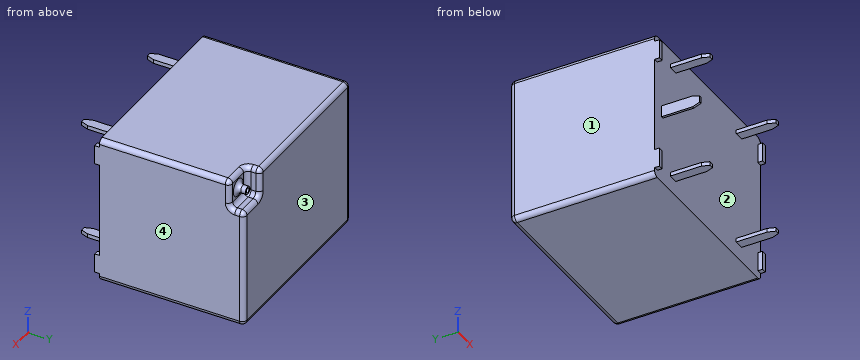
from build123d import *
from OCP.BRepFilletAPI import BRepFilletAPI_MakeChamfer

# Parameters (mm, degrees)
SKETCH_1_W          = 19.6
SKETCH_1_H          = 15.6
EXTRUDE_1_DEPTH     = 15.2
SKETCH_2_W          = 3
SKETCH_2_H          = 3
CUT_EXTRUDE_1_DEPTH = 1.5
SKETCH_3_R          = 0.4
SKETCH_3_R_2        = 0.25
EXTRUDE_2_DEPTH     = 1
SKETCH_5_W          = 0.5
SKETCH_5_H          = 2
EXTRUDE_4_DEPTH     = 0.5
FILLET_1_R          = 0.5
SKETCH_4_W          = 0.25
SKETCH_4_H          = 1.2
SKETCH_4_W_2        = 1
SKETCH_4_H_2        = 0.4
EXTRUDE_3_DEPTH     = 4
CHAMFER_1_SIZE      = 0.75
CHAMFER_1_SIZE2     = 0.272977676


with BuildPart() as part:
    # Эскиз1 → Бобышка-Вытянуть1 (new body)
    with BuildSketch(Plane(origin=(0, 0, 0), x_dir=(1, 0, 0), z_dir=(0, 1, 0))):
        Rectangle(SKETCH_1_W, SKETCH_1_H)
    extrude(amount=EXTRUDE_1_DEPTH)

    # Эскиз2 → Вырез-Вытянуть1 (cut)
    with BuildSketch(Plane(origin=(0, 15.2, 0), x_dir=(1, 0, 0), z_dir=(0, 1, 0))):
        with Locations((8.3, -6.3)):
            Rectangle(SKETCH_2_W, SKETCH_2_H)
    extrude(amount=-CUT_EXTRUDE_1_DEPTH, mode=Mode.SUBTRACT)

    # Эскиз3 → Бобышка-Вытянуть2 (add)
    with BuildSketch(Plane(origin=(0, 13.7, 0), x_dir=(1, 0, 0), z_dir=(0, 1, 0))):
        with Locations(Location((8.3, -6.3, 0), (0, 0, 270))):
            Circle(SKETCH_3_R)
        with Locations(Location((8.3, -6.3, 0), (0, 0, 270))):
            Circle(SKETCH_3_R_2, mode=Mode.SUBTRACT)
    extrude(amount=EXTRUDE_2_DEPTH)

    # Эскиз5 → Бобышка-Вытянуть4 (add)
    with BuildSketch(Plane.XZ):
        with Locations((-9.55, 6)):
            Rectangle(SKETCH_5_W, SKETCH_5_H)
        with Locations((-9.55, -6)):
            Rectangle(SKETCH_5_W, SKETCH_5_H)
        with Locations((9.55, -6)):
            Rectangle(SKETCH_5_W, SKETCH_5_H)
        with Locations((9.55, 6)):
            Rectangle(SKETCH_5_W, SKETCH_5_H)
    extrude(amount=EXTRUDE_4_DEPTH)

    # Скругление1
    fillet_1_edges = [part.edges().sort_by_distance(p)[0] for p in [
        (8.3, 15.2, 4.8),
        (-9.8, 7.6, -7.8),
        (-9.8, 15.2, 0),
        (9.8, 7.6, -7.8),
        (0, 15.2, -7.8),
        (9.8, 15.2, -1.5),
        (8.3, 13.7, 5.9),
        (6.8, 13.7, 6.3),
        (8.3, 13.7, 4.8),
        (9.8, 14.45, 4.8),
        (8.3, 13.7, 7.8),
        (9.8, 13.7, 6.3),
        (6.8, 14.45, 4.8),
        (6.8, 15.2, 6.3),
        (6.8, 14.45, 7.8),
        (-1.5, 15.2, 7.8),
        (9.8, 6.85, 7.8),
        (-9.8, 7.6, 7.8),
    ]]
    fillet(fillet_1_edges, radius=FILLET_1_R)

    # Эскиз4 → Бобышка-Вытянуть3 (add)
    with BuildSketch(Plane.XZ):
        with Locations((-8.4, 0)):
            Rectangle(SKETCH_4_W, SKETCH_4_H)
        with Locations((-6.4, 6)):
            Rectangle(SKETCH_4_W_2, SKETCH_4_H_2)
        with Locations((5.8, 6)):
            Rectangle(SKETCH_4_W_2, SKETCH_4_H_2)
        with Locations((5.8, -6)):
            Rectangle(SKETCH_4_W_2, SKETCH_4_H_2)
        with Locations((-6.4, -6)):
            Rectangle(SKETCH_4_W_2, SKETCH_4_H_2)
    extrude(amount=EXTRUDE_3_DEPTH)

    # Фаска1: one chamfer whose edges measure the first distance from different faces: ONE call of the kernel's chamfer builder (chamfer() names one face for all edges)
    chamfer_1_edges_1 = [part.edges().sort_by_distance(p)[0] for p in [
        (-8.4, -4, 0.6),
    ]]
    chamfer_1_side_1 = [part.faces().sort_by_distance(p)[0] for p in [
        (-8.4, -2, 0.6),
    ]]
    chamfer_1_edges_2 = [part.edges().sort_by_distance(p)[0] for p in [
        (-8.4, -4, -0.6),
    ]]
    chamfer_1_side_2 = [part.faces().sort_by_distance(p)[0] for p in [
        (-8.4, -2, -0.6),
    ]]
    chamfer_1_edges_3 = [part.edges().sort_by_distance(p)[0] for p in [
        (-6.9, -4, 6),
    ]]
    chamfer_1_side_3 = [part.faces().sort_by_distance(p)[0] for p in [
        (-6.9, -2, 6),
    ]]
    chamfer_1_edges_4 = [part.edges().sort_by_distance(p)[0] for p in [
        (-5.9, -4, 6),
    ]]
    chamfer_1_side_4 = [part.faces().sort_by_distance(p)[0] for p in [
        (-5.9, -2, 6),
    ]]
    chamfer_1_edges_5 = [part.edges().sort_by_distance(p)[0] for p in [
        (5.3, -4, 6),
    ]]
    chamfer_1_side_5 = [part.faces().sort_by_distance(p)[0] for p in [
        (5.3, -2, 6),
    ]]
    chamfer_1_edges_6 = [part.edges().sort_by_distance(p)[0] for p in [
        (6.3, -4, 6),
    ]]
    chamfer_1_side_6 = [part.faces().sort_by_distance(p)[0] for p in [
        (6.3, -2, 6),
    ]]
    chamfer_1_edges_7 = [part.edges().sort_by_distance(p)[0] for p in [
        (6.3, -4, -6),
    ]]
    chamfer_1_side_7 = [part.faces().sort_by_distance(p)[0] for p in [
        (6.3, -2, -6),
    ]]
    chamfer_1_edges_8 = [part.edges().sort_by_distance(p)[0] for p in [
        (5.3, -4, -6),
    ]]
    chamfer_1_side_8 = [part.faces().sort_by_distance(p)[0] for p in [
        (5.3, -2, -6),
    ]]
    chamfer_1_edges_9 = [part.edges().sort_by_distance(p)[0] for p in [
        (-5.9, -4, -6),
    ]]
    chamfer_1_side_9 = [part.faces().sort_by_distance(p)[0] for p in [
        (-5.9, -2, -6),
    ]]
    chamfer_1_edges_10 = [part.edges().sort_by_distance(p)[0] for p in [
        (-6.9, -4, -6),
    ]]
    chamfer_1_side_10 = [part.faces().sort_by_distance(p)[0] for p in [
        (-6.9, -2, -6),
    ]]
    chamfer_1 = BRepFilletAPI_MakeChamfer(part.part.solid().wrapped)
    for e in chamfer_1_edges_1:
        chamfer_1.Add(CHAMFER_1_SIZE, CHAMFER_1_SIZE2, e.wrapped, chamfer_1_side_1[0].wrapped)  # the first distance lies on this face
    for e in chamfer_1_edges_2:
        chamfer_1.Add(CHAMFER_1_SIZE, CHAMFER_1_SIZE2, e.wrapped, chamfer_1_side_2[0].wrapped)  # the first distance lies on this face
    for e in chamfer_1_edges_3:
        chamfer_1.Add(CHAMFER_1_SIZE, CHAMFER_1_SIZE2, e.wrapped, chamfer_1_side_3[0].wrapped)  # the first distance lies on this face
    for e in chamfer_1_edges_4:
        chamfer_1.Add(CHAMFER_1_SIZE, CHAMFER_1_SIZE2, e.wrapped, chamfer_1_side_4[0].wrapped)  # the first distance lies on this face
    for e in chamfer_1_edges_5:
        chamfer_1.Add(CHAMFER_1_SIZE, CHAMFER_1_SIZE2, e.wrapped, chamfer_1_side_5[0].wrapped)  # the first distance lies on this face
    for e in chamfer_1_edges_6:
        chamfer_1.Add(CHAMFER_1_SIZE, CHAMFER_1_SIZE2, e.wrapped, chamfer_1_side_6[0].wrapped)  # the first distance lies on this face
    for e in chamfer_1_edges_7:
        chamfer_1.Add(CHAMFER_1_SIZE, CHAMFER_1_SIZE2, e.wrapped, chamfer_1_side_7[0].wrapped)  # the first distance lies on this face
    for e in chamfer_1_edges_8:
        chamfer_1.Add(CHAMFER_1_SIZE, CHAMFER_1_SIZE2, e.wrapped, chamfer_1_side_8[0].wrapped)  # the first distance lies on this face
    for e in chamfer_1_edges_9:
        chamfer_1.Add(CHAMFER_1_SIZE, CHAMFER_1_SIZE2, e.wrapped, chamfer_1_side_9[0].wrapped)  # the first distance lies on this face
    for e in chamfer_1_edges_10:
        chamfer_1.Add(CHAMFER_1_SIZE, CHAMFER_1_SIZE2, e.wrapped, chamfer_1_side_10[0].wrapped)  # the first distance lies on this face
    add(Compound.cast(chamfer_1.Shape()), mode=Mode.REPLACE)


solid = part.part
Input: part model. Units: mm. Frame: model coordinates. Face numbers are marked on the shaded views. Coordinates: 2 decimals unless noted, no trailing zeros. Loops run counter-clockwise (first coordinate to the right, second up) from the corner with the lowest first, then second, coordinate; pieces in that order, holes last.
(1) Section B-B on z = 3.5. Return the cut outline in (x, y).
(2) First-contact query: pin 1 Ø0.5 at (x, y) = (-6.5, -1.5) entering from +Z; pin 2 Ø1.5 at (y, z) = (-1, -1) entering from +X (3 decimals); pin 3 Ø2 at (x, z) = (-4, -0.5) entering from -Y. Flat tips, straight axial feed; report the tip coordinate or a pass-through.
(3) Pull-direction query (X, two-part tool) for the marked faces 1, 2, 3 and 4; classes: released by +X, released by -X, zero draft, split by the parting line, or undercut.
(4) Section D-D on z = -6.5. Return the cut outline in (x, y).
(5) Material intervals for probe 1 along Y at (x, z) = (-5.5, 1.75); probe 2 along X at (y, z) = (14.1, 6.3); probe 3 along X at (y, z) = (13.95, 6.3), sorted ascending.
(6) Section A-A on y = -2. Return the cut outline in (x, z) (3 decimals).
(7) Section C-C on x = 4. Return the cut outline in (y, z), then the cut area to 3 significant figures.
Data:
1. outline: (-9.8, 0) - (9.8, 0) - (9.8, 14.7) arc R0.5 ccw to (9.3, 15.2) - (-9.3, 15.2) arc R0.5 ccw to (-9.8, 14.7) - close
2. pin 1: stops at z = 6.2
2. pin 2: stops at x = -8.275
2. pin 3: stops at y = 0
3. face 1: released by -X
3. face 2: undercut
3. face 3: zero draft
3. face 4: released by +X
4. outline: (-9.8, -0.5) - (-9.3, -0.5) - (-9.3, 0) - (9.3, 0) - (9.3, -0.5) - (9.8, -0.5) - (9.8, 14.7) arc R0.5 ccw to (9.3, 15.2) - (-9.3, 15.2) arc R0.5 ccw to (-9.8, 14.7) - close
5. probe 1: y = 0 to 15.2
5. probe 2: x = -9.8 to 6.81, 7.89 to 8.05, 8.55 to 8.71
5. probe 3: x = -9.8 to 6.87, 7.83 to 8.05, 8.55 to 8.77
6. outline: (-8.525, -0.6) - (-8.275, -0.6) - (-8.275, 0.6) - (-8.525, 0.6) - close; (-6.9, -6.2) - (-5.9, -6.2) - (-5.9, -5.8) - (-6.9, -5.8) - close; (-6.9, 5.8) - (-5.9, 5.8) - (-5.9, 6.2) - (-6.9, 6.2) - close; (5.3, -6.2) - (6.3, -6.2) - (6.3, -5.8) - (5.3, -5.8) - close; (5.3, 5.8) - (6.3, 5.8) - (6.3, 6.2) - (5.3, 6.2) - close
7. outline: (0, -7.8) - (14.7, -7.8) arc R0.5 ccw to (15.2, -7.3) - (15.2, 7.3) arc R0.5 ccw to (14.7, 7.8) - (0, 7.8) - close
7. area: 237 mm2
